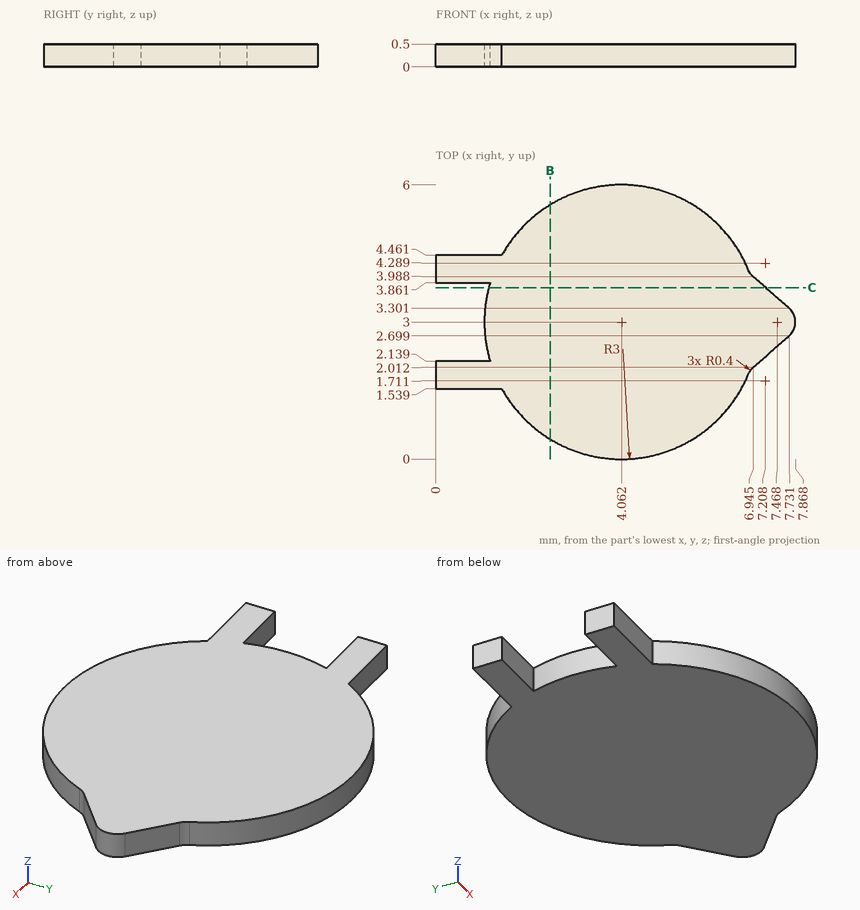
Can you work these out from the drawing? Everything is in mm from the part's minimum corner. Give positions to 0.01 mm unless a question says otherwise; leave off trailing zeros. Order: outer loops, then holes, each group sorted by start corner. A loop starts at its lowest first (then second) coordinate and runs counter-clockwise, first axis right, second up. Notation, with made-up numbers: M -29.5,-18.75 L 13.5,-18.75 A7 cw 13.5,-11.75 Z; hole C 82,-29 d11. An arc over 180 degrees is marked long. Use a Markdown table: item, result. Add a question column.
Item 1: If I drill on L1, parallel to Y at x = 1, z = 0.35; L2, parallel to X at y = 5, z = 0.1 (1 decimal); L3, parallel to Y at x = 1.75, z = 0.2 (1 decimal), over which ranges is the centre line in solid material (lowest first)? Write a range as [from, to].
Item 2: Suppose I cut it at B-B (x = 2.5). List the corners of the cut face in (y, z) for me.
Item 3: Suppose I cut it at C-C (y = 3.75). List the corners of the cut face in (x, z) for me.
Answer sheet:
| question | item | result |
|---|---|---|
| 1 | L1 | y = [1.54, 2.14], [3.86, 4.46] |
| 1 | L2 | x = [1.8, 6.3] |
| 1 | L3 | y = [1.1, 4.9] |
| 2 | outline | M 0.44,0 L 5.56,0 L 5.56,0.5 L 0.44,0.5 Z |
| 3 | outline | M 1.16,0 L 7.22,0 L 7.22,0.5 L 1.16,0.5 Z |
